Check sheet for the modelled part. Datum: model origin and axes. Units: mm. A direction names the side the tool comes from. Give positions to 0.01 mm unless a question says otherwise; leave off trailing zeros. Loops run counter-clockwise (first coordinate to the right, second up) from the corner with the lowest first, then second, coordinate; pieces in that order, holes last. Notation, with made-up numbers: M -28,43 L 25,43 A16 cw 25,59 Z; hole C -33.5,9 d1. An arc over 180 degrees is marked long. Write each question's results on one line, items separated by ' | '. Start each with the question number.
1. Sectioned sample at A-A on y = 22.75. Record the cut outline in (x, z), and give its area (3 significant figures).
2. Sectioned sample at B-B on x = -35. Record the cut outline in (y, z), and give its area (4 significant figures).
3. Material ranges on line 1 along X through (y, z) = (1.65, 8.7); line 2 along Z through (x, y) = (37.5, 18.25); line 3 along Y through (x, z) = (-7, 8), recorded low to high.
4. Go/stop test with flat-tipped pins: pin 1 (6 mm diameter, centred on x = 28, y = 16.5, fed in from +Z); pin 2 (2.5 mm diameter, centred on y = 1.5, z = 0, fed in from -X); pin 3 (10 mm diameter, centred on x = 27.5, y = 11.5, fed in from -Z). Record where each tip stops, or that it passes through.
5. Tool access check on faces 4 (the cylindrical face through (33.636, 20.75, -0.965)), 5 (the cylindrical face through (-17.746, 4.014, 9.738)). Record the directions out of +Z, -Z, +X, -X, +Y, -Y that give a thin tool (end or side, any length) a straight path to the whole face; none if there is none.
6. Sectioned sample at D-D on x = -25. Record the cut outline in (y, z).
7. Draft check along Z on faces 1 (the flat face through (-28, 15, -3.5)), 2 (the flat face through (15, 3, -5)), 3 (the flat face through (-40, 21, -1)). Enter one of: pulls with the +Z half, pulls with the -Z half, needs draft (parallel to the pull), parting line crosses it, or undercut.
8. Sectioned sample at C-C on x = 15.75. Record the cut outline in (y, z), and give its area (3 significant figures).
```python
from build123d import *

# Parameters (mm, degrees)
SKETCH1_W           = 60
SKETCH1_H           = 23
BOSS_EXTRUDE1_DEPTH = 5
BOSS_EXTRUDE2_START = -10
SKETCH2_R           = 1.85
BOSS_EXTRUDE2_DEPTH = 5
SKETCH3_R           = 1.35
CUT_EXTRUDE1_DEPTH  = 49.295962564
SKETCH4_R           = 2.25
CUT_EXTRUDE2_DEPTH  = 2
FILLET1_R           = 3


with BuildPart() as part:
    # Sketch1 → Boss-Extrude1 (new body)
    with BuildSketch(Plane(origin=(0, 0, 0), x_dir=(1, 0, 0), z_dir=(0, 1, 0))):
        Rectangle(SKETCH1_W, SKETCH1_H)
    extrude(amount=BOSS_EXTRUDE1_DEPTH)

    # Sketch2 → Boss-Extrude2 (add)
    # profile 1 of 2: a face of its own
    with BuildSketch(Plane.XY.offset(11.5).offset(BOSS_EXTRUDE2_START)):
        Polygon((-40, 16.5), (-30, 5), (-16.521636852, 5), (-16.521636852, 24.5), (-40, 24.5), align=None)
        with Locations((-35, 19.5)):
            Circle(SKETCH2_R, mode=Mode.SUBTRACT)
        with Locations((-22, 19.5)):
            Circle(SKETCH2_R, mode=Mode.SUBTRACT)
    # profile 2 of 2: a face of its own
    with BuildSketch(Plane.XY.offset(11.5).offset(BOSS_EXTRUDE2_START)):
        Polygon((40, 16.5), (40, 24.5), (16.521636852, 24.5), (16.521636852, 5), (30, 5), align=None)
        with Locations((22, 19.5)):
            Circle(SKETCH2_R, mode=Mode.SUBTRACT)
        with Locations((35, 19.5)):
            Circle(SKETCH2_R, mode=Mode.SUBTRACT)
    extrude(amount=-BOSS_EXTRUDE2_DEPTH)

    # Sketch3 → Cut-Extrude1 (cut, through all)
    with BuildSketch(Plane.XZ):
        with Locations(Location((-15.75, 8.7, 0), (0, 0, 270))):
            Circle(SKETCH3_R)
        with Locations(Location((15.75, 8.7, 0), (0, 0, 270))):
            Circle(SKETCH3_R)
        with Locations(Location((15.75, -6.34, 0), (0, 0, 270))):
            Circle(SKETCH3_R)
        with Locations(Location((-15.75, -6.34, 0), (0, 0, 270))):
            Circle(SKETCH3_R)
    extrude(amount=-CUT_EXTRUDE1_DEPTH, mode=Mode.SUBTRACT)

    # Sketch4 → Cut-Extrude2 (cut)
    with BuildSketch(Plane(origin=(0, 5, 0), x_dir=(1, 0, 0), z_dir=(0, 1, 0))):
        with Locations(Location((-15.75, 6.34, 0), (0, 0, 270))):
            Circle(SKETCH4_R)
        with Locations(Location((15.75, 6.34, 0), (0, 0, 270))):
            Circle(SKETCH4_R)
        with Locations(Location((15.75, -8.7, 0), (0, 0, 270))):
            Circle(SKETCH4_R)
        with Locations(Location((-15.75, -8.7, 0), (0, 0, 270))):
            Circle(SKETCH4_R)
    extrude(amount=-CUT_EXTRUDE2_DEPTH, mode=Mode.SUBTRACT)

    # Fillet1
    fillet1_edges = [part.edges().sort_by_distance(p)[0] for p in [
        (30, 2.5, 11.5),
        (-30, 2.5, 11.5),
        (-30, 2.5, -11.5),
        (30, 2.5, -11.5),
    ]]
    fillet(fillet1_edges, radius=FILLET1_R)


solid = part.part
```
Output values:
1) outline: M -40,-3.5 L -16.52,-3.5 L -16.52,1.5 L -40,1.5 Z; M 16.52,-3.5 L 40,-3.5 L 40,1.5 L 16.52,1.5 Z | area: 235 mm2
2) outline: M 10.75,-3.5 L 17.65,-3.5 L 17.65,1.5 L 10.75,1.5 Z; M 21.35,-3.5 L 24.5,-3.5 L 24.5,1.5 L 21.35,1.5 Z | area: 50.25 mm2
3) line 1: -29.99 to -17.1, -14.4 to 14.4, 17.1 to 29.99 | line 2: -3.5 to 1.5 | line 3: 0 to 5
4) pin 1: z = 1.5 | pin 2: x = -30 | pin 3: z = -3.5
5) face 4: +Z, -Z | face 5: +Y
6) outline: M 0,-11.5 L 5,-11.5 L 5,-3.5 L 24.5,-3.5 L 24.5,1.5 L 5,1.5 L 5,11.5 L 0,11.5 Z
7) face 1: pulls with the -Z half | face 2: undercut | face 3: needs draft
8) outline: M 0,-11.5 L 5,-11.5 L 5,-8.59 L 3,-8.59 L 3,-7.69 L 0,-7.69 Z; M 0,-4.99 L 3,-4.99 L 3,-4.09 L 5,-4.09 L 5,6.45 L 3,6.45 L 3,7.35 L 0,7.35 Z; M 0,10.05 L 3,10.05 L 3,10.95 L 5,10.95 L 5,11.5 L 0,11.5 Z | area: 80.8 mm2
